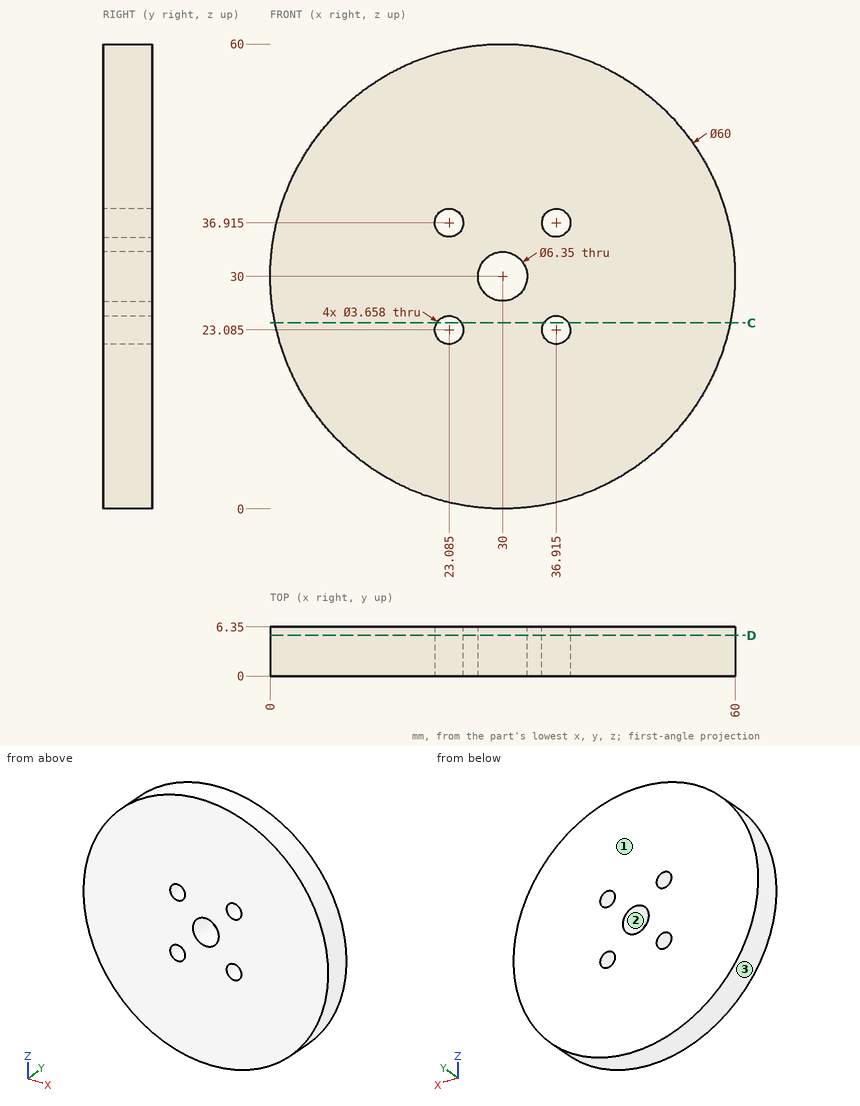
The drawing under review shows one solid part. Ordinate dimensions are in mm from its lowest x, y, z. Coordinates: 2 decimals unless noted, no trailing zeros. Write each loop counter-clockwise with the first axis right and the second up, starting at its lowest first coordinate (ties: lowest second). Pieces come first, ordered by that corner, then holes. Notation, with made-up numbers: (-37, 14.5) -> (2, 14.5) arc R22 cw to (2, 43.5) -> close; hole circle Ø5 at (19.5, -34.75). An arc over 180 degrees is marked (long way). One line per item, written item: value. Start each with the question number.
Q1. Clearance check with flat-ended pins moving along their axes: P1, Ø1.5, axis at y = 2.5, z = 27, coming from the +X side (1 decimal); P2, Ø1.5, axis at x = 38.5, y = 3, coming from the +Z side; P3, Ø2, axis at x = 38, y = 3.5, coming from the +Z side. State where each tip first meets the part, or that it passes through.
Q2. Add section C-C, the plane z = 24. Give the boundary of the cut face in (x, y).
Q3. The part is to be moulded in two halves that separate along Z. For the marked faces 1, 2 and 3, say which applies: +Z half, -Z half, draft (parallel to the pull), parting line (faces both ways), or undercut.
Q4. Add section D-D, the plane y = 5.25. Count the separate pieces of the cut face and the enclosed holes in it, then the cut area to 3 significant figures.
Q5. To check wall thickness, follow probe 1 along X at (y, z) = (3.25, 30) (1 decimal); probe 2 along Z at (x, y) = (37.5, 3.25); probe 3 along Z at (x, y) = (36, 5) (1 decimal). State the ranges of each line that lie inside material, in increasing order.
Response:
1. P1: x = 59.9
1. P2: z = 58.98
1. P3: z = 59.17
2. outline: (0.61, 0) -> (21.5, 0) -> (21.5, 6.35) -> (0.61, 6.35) -> close; (24.67, 0) -> (35.33, 0) -> (35.33, 6.35) -> (24.67, 6.35) -> close; (38.5, 0) -> (59.39, 0) -> (59.39, 6.35) -> (38.5, 6.35) -> close
3. face 1: draft
3. face 2: undercut
3. face 3: parting line
4. separate pieces: 1
4. enclosed holes: 5
4. area: 2,750 mm²
5. probe 1: 0 to 26.8, 33.2 to 60
5. probe 2: 0.95 to 21.35, 24.82 to 35.18, 38.65 to 59.05
5. probe 3: 0.6 to 21.5, 24.7 to 35.3, 38.5 to 59.4
